from build123d import *

# Parameters (mm, degrees)
SKETCH_1_W          = 19.8
SKETCH_1_H          = 9.8
EXTRUDE_1_DEPTH     = 1.8
SKETCH_2_W          = 15
SKETCH_2_H          = 8
EXTRUDE_2_DEPTH     = 6
SKETCH_3_W          = 1
SKETCH_3_H          = 3
CUT_EXTRUDE_1_DEPTH = 3
SKETCH_4_W          = 19.16
SKETCH_4_H          = 0.95
CUT_EXTRUDE_2_DEPTH = 3
SKETCH_7_W          = 1
SKETCH_7_H          = 3
CUT_EXTRUDE_4_DEPTH = 3


with BuildPart() as part:
    # 草图1 → 凸台-拉伸1 (new body)
    with BuildSketch(Plane(origin=(0, 0, 0), x_dir=(1, 0, 0), z_dir=(0, 1, 0))):
        with Locations((-9.9, 4.9)):
            Rectangle(SKETCH_1_W, SKETCH_1_H)
    extrude(amount=EXTRUDE_1_DEPTH)

    # 草图2 → 凸台-拉伸2 (add)
    with BuildSketch(Plane(origin=(0, 1.8, 0), x_dir=(1, 0, 0), z_dir=(0, 1, 0))):
        with Locations((-9.9, 4.7)):
            Rectangle(SKETCH_2_W, SKETCH_2_H)
    extrude(amount=EXTRUDE_2_DEPTH)

    # 草图3 → 切除-拉伸1 (cut)
    with BuildSketch(Plane(origin=(0, 1.8, 0), x_dir=(1, 0, 0), z_dir=(0, 1, 0))):
        with Locations((-19.3, 8.3)):
            Rectangle(SKETCH_3_W, SKETCH_3_H)
    extrude(amount=-CUT_EXTRUDE_1_DEPTH, mode=Mode.SUBTRACT)

    # 草图4 → 切除-拉伸2 (cut)
    with BuildSketch(Plane(origin=(0, 1.8, 0), x_dir=(1, 0, 0), z_dir=(0, 1, 0))):
        with Locations((-9.58, 9.460376994)):
            Rectangle(SKETCH_4_W, SKETCH_4_H)
    extrude(amount=-CUT_EXTRUDE_2_DEPTH, mode=Mode.SUBTRACT)

    # 草图7 → 切除-拉伸4 (cut)
    with BuildSketch(Plane(origin=(0, 1.8, 0), x_dir=(1, 0, 0), z_dir=(0, 1, 0))):
        with Locations((-0.5, 7.485376994)):
            Rectangle(SKETCH_7_W, SKETCH_7_H)
    extrude(amount=-CUT_EXTRUDE_4_DEPTH, mode=Mode.SUBTRACT)


solid = part.part
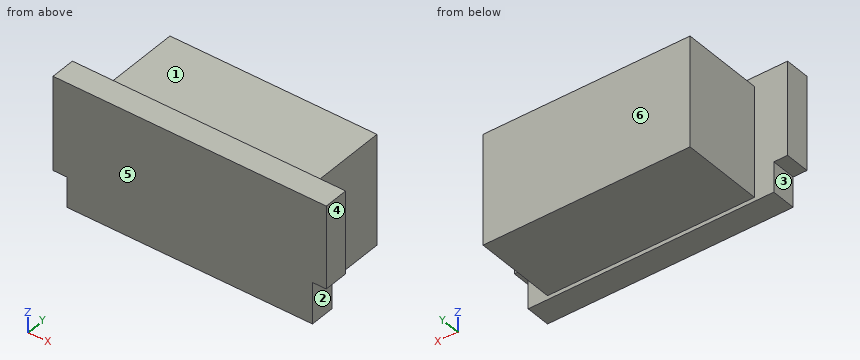
The model under review builds one solid part; all positions refer to its coordinate system, in mm. Face numbers are marked on the shaded views. A direction names the side the tool comes from. Give positions to 0.01 mm unless a question says otherwise; leave off trailing zeros. Loops run counter-clockwise (first coordinate to the right, second up) from the corner with the lowest first, then second, coordinate; pieces in that order, holes last. Notation, with made-up numbers: (-30, 70) -> (23, 70) arc R11 cw to (23, 89) -> close; hole circle Ø10 at (89, 62.25). An arc over 180 degrees is marked (long way). Write each question's results on one line, items separated by ' | '.
1) Tool access review of the marked faces 1, 2 and 3: name each direction out of +Z, -Z, +X, -X, +Y, -Y from which nothing blocks a thin tool from reaching the whole face with its end or side.
Conclusion:
face 1: +Z, +X, -X, +Y | face 2: -Z, +X, +Y, -Y | face 3: -Z, -X, +Y, -Y
2) Take a section at C-C, the plane x = -18.25. Give the boundary of the cut face in (y, z), plus the area to 3 significant figures.
Conclusion:
outline: (0, -8.99) -> (1.8, -8.99) -> (1.8, 0) -> (0, 0) -> close | area: 16.2 mm^2
3) Take a section at A-A, the plane y = 1. Give the boundary of the cut face in (x, z), plus the area to 3 significant figures.
Conclusion:
outline: (-19.8, -6.8) -> (-18.8, -6.8) -> (-18.8, -8.99) -> (-1, -8.99) -> (-1, -5.99) -> (0, -5.99) -> (0, 0) -> (-19.8, 0) -> close | area: 173 mm^2
4) For line 1 along Z through (x, y) = (-10.5, 4.5); line 2 along X through (y, z) = (3.5, -5); line 3 along Y through (x, z) = (-18, -4.75), list the stretches that pass through material, from the lowest coordinate up. Write a range as from..to.
Conclusion:
line 1: z = -8.7..-0.7 | line 2: x = -17.4..-2.4 | line 3: y = 0..1.8
5) Take a section at D-D, the plane z = -0.5. Give the boundary of the cut face in (x, y).
Conclusion:
outline: (-19.8, 0) -> (0, 0) -> (0, 1.8) -> (-19.8, 1.8) -> close
6) Draft analysis for pull direction Y (two halves, no side actions). For the marked faces 4, 5 and 6, state which applies: pulls with the +Y half, pulls with the -Y half, needs draft (parallel to the pull), parting line crosses it, or undercut.
Conclusion:
face 4: needs draft | face 5: pulls with the -Y half | face 6: pulls with the +Y half
7) Take a section at B-B, the plane z = -4.75. Give the boundary of the cut face in (x, y).
Conclusion:
outline: (-19.8, 0) -> (0, 0) -> (0, 1.8) -> (-2.4, 1.8) -> (-2.4, 7.8) -> (-17.4, 7.8) -> (-17.4, 1.8) -> (-19.8, 1.8) -> close
8) Insertion check: pin 1 Ø0.8 at (x, y) = (-0.5, 0.5) entering from -Z; pin 2 Ø2 at (y, z) = (1, -8.5) entering from -X; pin 3 Ø1.5 at (x, y) = (-17.5, 3.5) entering from +Z. Each pin has a flat end and moves straight along its axis. Give the tip position at first contact, or say it passes through.
Conclusion:
pin 1: stops at z = -5.99 | pin 2: stops at x = -18.8 | pin 3: stops at z = -0.7
